```python
from build123d import *

# Parameters (mm, degrees)
SKETCH2_W           = 35
SKETCH2_H           = 3
BOSS_EXTRUDE1_DEPTH = 90
CUT_EXTRUDE1_START  = -13
SKETCH3_R           = 1.25
CUT_EXTRUDE1_DEPTH  = 14
SKETCH4_R           = 2.25
CUT_EXTRUDE2_DEPTH  = 2


with BuildPart() as part:
    # Sketch2 → Boss-Extrude1 (new body)
    with BuildSketch(Plane.XY):
        Polygon((17.5, 10.5), (17.5, 1.5), (17.5, -1.5), (20.5, -1.5), (20.5, 10.5), align=None)
        Rectangle(SKETCH2_W, SKETCH2_H)
        Polygon((-17.5, -1.5), (-17.5, 1.5), (-17.5, 10.5), (-20.5, 10.5), (-20.5, -1.5), align=None)
    boss_extrude1 = extrude(amount=BOSS_EXTRUDE1_DEPTH)

    # Sketch3 → Cut-Extrude1 (cut)
    with BuildSketch(Plane.XZ.offset(1.5).offset(CUT_EXTRUDE1_START)):
        with Locations((-8, 83)):
            Circle(SKETCH3_R)
        with Locations((8, 83)):
            Circle(SKETCH3_R)
        with Locations((8, 51)):
            Circle(SKETCH3_R)
        with Locations((-8, 51)):
            Circle(SKETCH3_R)
    cut_extrude1 = extrude(amount=CUT_EXTRUDE1_DEPTH, mode=Mode.SUBTRACT)

    # Sketch4 → Cut-Extrude2 (cut)
    with BuildSketch(Plane.XZ.offset(1.5)):
        with Locations((-8, 83)):
            Circle(SKETCH4_R)
        with Locations((8, 83)):
            Circle(SKETCH4_R)
        with Locations((8, 51)):
            Circle(SKETCH4_R)
        with Locations((-8, 51)):
            Circle(SKETCH4_R)
    cut_extrude2 = extrude(amount=-CUT_EXTRUDE2_DEPTH, mode=Mode.SUBTRACT)

    # Mirror1: Boss-Extrude1, Cut-Extrude1, Cut-Extrude2 across plane
    add(boss_extrude1.mirror(Plane.XY))
    add(cut_extrude1.mirror(Plane.XY), mode=Mode.SUBTRACT)
    add(cut_extrude2.mirror(Plane.XY), mode=Mode.SUBTRACT)


solid = part.part
```
Input: part model. Units: mm. Frame: model coordinates. A direction names the side the tool comes from. Give positions to 0.01 mm unless a question says otherwise; leave off trailing zeros. Order: outer loops, then holes, each group sorted by start corner. A loop starts at its lowest first (then second) coordinate and runs counter-clockwise, first axis right, second up. Notation, with made-up numbers: (2.5, 79) - (48.5, 79) arc R25 ccw to (48.5, 113) - close; hole circle Ø9 at (40, 47.25). An arc over 180 degrees is marked (long way). Use a Markdown table: item, result.
(1) Section query A-A (y = 6.75). Output: boundary loops of the cut face in (x, z).
Computed values:
| item | result |
|---|---|
| outline | (-20.5, -90) - (-17.5, -90) - (-17.5, 90) - (-20.5, 90) - close; (17.5, -90) - (20.5, -90) - (20.5, 90) - (17.5, 90) - close |
(2) Access query for faces 5 (the cylindrical face through (7.512, -0.514, 80.804)), 6 (the flat face through (20.5, 4, 1)), 7 (the flat face through (-17.5, 6, 1)). Directions: +Z, -Z, +X, -X, +Y, -Y. A direction counts if a zero-diameter tool reaches every point of the face in a straight line with its end or side. Return the directions, or none.
Computed values:
| item | result |
|---|---|
| face 5 | -Y |
| face 6 | +Z, -Z, +X, +Y, -Y |
| face 7 | +Z, -Z, +Y |
(3) Pin query (flat end, axial travel): pin 1 (17.5 mm diameter, centred on x = -6.5, z = -14, fed in from +Y); pin 2 (2 mm diameter, centred on x = -9, z = 83, fed in from -Y). Return the tip coordinate at first contact, or that it passes through.
Computed values:
| item | result |
|---|---|
| pin 1 | stops at y = 1.5 |
| pin 2 | stops at y = 0.5 |
(4) Line query: line 1 (Z direction, x = -8, y = -0.45); line 2 (X direction, y = 0.75, z = -83); line 3 (X direction, y = 9.75, z = -52). Output: solid intervals per line, ascending. Write a range as from..to.
Computed values:
| item | result |
|---|---|
| line 1 | z = -90..-85.25, -80.75..-53.25, -48.75..48.75, 53.25..80.75, 85.25..90 |
| line 2 | x = -20.5..-9.25, -6.75..6.75, 9.25..20.5 |
| line 3 | x = -20.5..-17.5, 17.5..20.5 |
(5) Section query C-C (x = -2.5). Output: boundary loops of the cut face in (y, z).
Computed values:
| item | result |
|---|---|
| outline | (-1.5, -90) - (1.5, -90) - (1.5, 90) - (-1.5, 90) - close |
(6) Draft query along Z for faces 1 (the flat face through (9, 0.5, 82)), 2 (the flat face through (0, 1, -90)), 3 (the flat face through (-19, 10.5, 1)), 4 (the flat face through (0, 1, 90)). Return one class per face: released by +Z, released by -Z, zero draft, split by the parting line, or undercut.
Computed values:
| item | result |
|---|---|
| face 1 | undercut |
| face 2 | released by -Z |
| face 3 | zero draft |
| face 4 | released by +Z |
(7) Section query B-B (z = -60). Output: boundary loops of the cut face in (x, y).
Computed values:
| item | result |
|---|---|
| outline | (-20.5, -1.5) - (20.5, -1.5) - (20.5, 10.5) - (17.5, 10.5) - (17.5, 1.5) - (-17.5, 1.5) - (-17.5, 10.5) - (-20.5, 10.5) - close |
